```python
from build123d import *

# Parameters (mm, degrees)
ESQUISSE1_R        = 10
BOSS_EXTRU_1_DEPTH = 20
CONG_1_R           = 25


with BuildPart() as part:
    # Esquisse1 → Boss.-Extru.1 (new body)
    with BuildSketch(Plane.XY):
        Polygon((25, 162.5), (-25, 162.5), (-25, -162.5), (25, -162.5), (45, -152.5), (25, -142.5), (45, -132.5), (25, -122.5), (45, -112.5), (25, -102.5), (45, -92.5), (25, -82.5), (45, -72.5), (25, -62.5), (45, -52.5), (25, -42.5), (45, -32.5), (25, -22.5), (45, -12.5), (25, -2.5), align=None)
        with Locations((0, 37.5)):
            Circle(ESQUISSE1_R, mode=Mode.SUBTRACT)
        with Locations((0, 137.5)):
            Circle(ESQUISSE1_R, mode=Mode.SUBTRACT)
    extrude(amount=BOSS_EXTRU_1_DEPTH)

    # Congé1
    cong_1_edges = [part.edges().sort_by_distance(p)[0] for p in [
        (-25, -162.5, 10),
        (25, 162.5, 10),
        (-25, 162.5, 10),
    ]]
    fillet(cong_1_edges, radius=CONG_1_R - 0.0001)  # a hair under: the kernel refuses the full size


solid = part.part
```
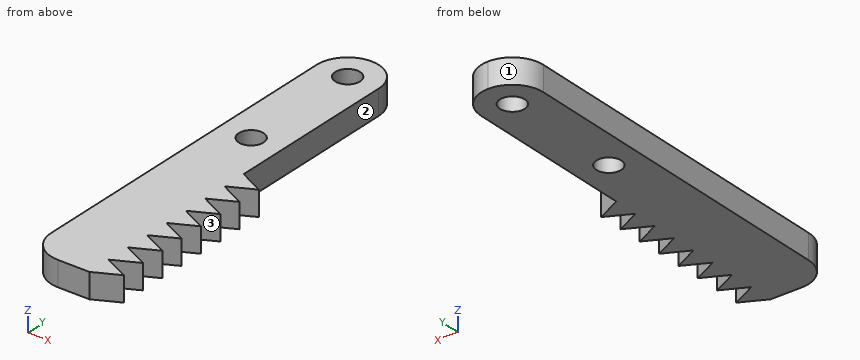
Verification items for the finished model (mm, model axes). Face numbers are marked on the shaded views. A direction names the side the tool comes from. Round coordinates to 2 decimals unless told otherwise and drop trailing zeros. Write each loop counter-clockwise with the first axis right and the second up, starting at its lowest first coordinate (ties: lowest second). Pieces come first, ordered by that corner, then holes.
1. Section check D-D on x = -3.5. Enter the section's corners in (y, z).
2. Section check A-A on x = 40.5. State how many separate pieces and enclosed holes the cut face has, plus the area to 3 significant figures.
3. Scan lines: L1, parallel to Y at x = 0, z = 13.5; L2, parallel to Y at x = 6.5, z = 2.25; L3, parallel to X at y = 63, z = 5.5. Record each from-to range of solid material in increasing order.
4. Access from +Z, -Z, +X, -X, +Y, -Y to the whole of each face (thin tool, end or side, straight path). Record for the marked faces 1, 2 and 3.
5. Section check B-B on y = 131.5. Enter the section's corners in (x, z), plus the area to 3 significant figures.
6. Gauge pin test, flat ends, axial feed: P1, Ø3, axis at y = 41.5, z = 13.5, coming from the +X side; P2, Ø3, axis at x = 11, z = 10, coming from the +Y side; P3, Ø1, axis at y = -78, z = 11, coming from the +X side. Record the tip position at first contact, or that the pin passes through.
Answer:
1. outline: (-162.25, 0) - (28.13, 0) - (28.13, 20) - (-162.25, 20) - close; (46.87, 0) - (128.13, 0) - (128.13, 20) - (46.87, 20) - close; (146.87, 0) - (162.25, 0) - (162.25, 20) - (146.87, 20) - close
2. separate pieces: 8
2. enclosed holes: 0
2. area: 720 mm2
3. L1: y = -162.5 to 27.5, 47.5 to 127.5, 147.5 to 162.5
3. L2: y = -162.5 to 29.9, 45.1 to 129.9, 145.1 to 161.64
3. L3: x = -25 to 25
4. face 1: +Z, -Z, -X, +Y
4. face 2: +Z, -Z, +X, +Y
4. face 3: +Z, -Z, +X
5. outline: (-25, 0) - (-8, 0) - (-8, 20) - (-25, 20) - close; (8, 0) - (25, 0) - (25, 20) - (8, 20) - close
5. area: 680 mm2
6. P1: stops at x = 25
6. P2: stops at y = 160.62
6. P3: stops at x = 35
